Check sheet for the modelled part. Datum: model origin and axes. Units: mm. Face numbers are marked on the shaded views. A direction names the side the tool comes from. Coordinates: 2 decimals unless noted, no trailing zeros. Write each loop counter-clockwise with the first axis right and the second up, starting at its lowest first coordinate (ties: lowest second). Pieces come first, ordered by that corner, then holes. Notation, with made-up numbers: M 43.25,65 L 70.25,65 A15 ccw 70.25,75 Z; hole C 38,-5 d1. An arc over 180 degrees is marked long. Answer as CSV lines item,"result".
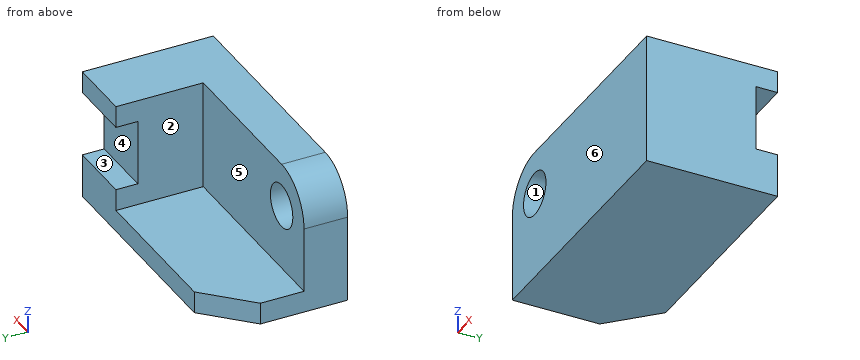
from build123d import *

# Parameters (mm, degrees)
SKETCH2_W           = 120
SKETCH2_H           = 60
BOSS_EXTRUDE1_DEPTH = 20
BOSS_EXTRUDE2_DEPTH = 40
FILLET1_R           = 20
CHAMFER1_SIZE       = 20
SKETCH8_W           = 30
SKETCH8_H           = 30
CUT_EXTRUDE1_DEPTH  = 10
SKETCH11_R          = 10
CUT_EXTRUDE3_DEPTH  = 141


with BuildPart() as part:
    # Sketch2 → Boss-Extrude1 (new body)
    with BuildSketch(Plane(origin=(0, 0, 0), x_dir=(1, 0, 0), z_dir=(0, 1, 0))):
        with Locations((-60, -30)):
            Rectangle(SKETCH2_W, SKETCH2_H)
    extrude(amount=-BOSS_EXTRUDE1_DEPTH)

    # Sketch3 → Boss-Extrude2 (add)
    with BuildSketch(Plane(origin=(0, 0, 0), x_dir=(1, 0, 0), z_dir=(0, 1, 0))):
        Polygon((-120, -10), (-30, -10), (-30, -60), (0, -60), (0, 0), (-120, 0), align=None)
    extrude(amount=BOSS_EXTRUDE2_DEPTH)

    # Fillet1
    fillet1_edges = [part.edges().sort_by_distance(p)[0] for p in [
        (-120, -10, 60),
    ]]
    fillet(fillet1_edges, radius=FILLET1_R)

    # Chamfer1
    chamfer1_edges = [part.edges().sort_by_distance(p)[0] for p in [
        (-120, 40, 5),
    ]]
    chamfer(chamfer1_edges, length=CHAMFER1_SIZE)

    # Sketch8 → Cut-Extrude1 (cut)
    with BuildSketch(Plane(origin=(0, 40, 0), x_dir=(1, 0, 0), z_dir=(0, 1, 0))):
        with Locations((-15, -35)):
            Rectangle(SKETCH8_W, SKETCH8_H)
    extrude(amount=-CUT_EXTRUDE1_DEPTH, mode=Mode.SUBTRACT)

    # Sketch11 → Cut-Extrude3 (cut, through all)
    with BuildSketch(Plane(origin=(0, 0, 0), x_dir=(1, 0, 0), z_dir=(0, 1, 0))):
        with Locations(Location((-100, -40, 0), (0, 0, 270))):
            Circle(SKETCH11_R)
    extrude(amount=-CUT_EXTRUDE3_DEPTH, mode=Mode.SUBTRACT)


solid = part.part
1) Section check C-C, the plane x = -15.5. Record the boundary of the cut face in (y, z), plus the area to 3 significant figures.
Answer key:
outline,"M -20,0 L 40,0 L 40,20 L 30,20 L 30,50 L 40,50 L 40,60 L -20,60 Z"
area,"3,300 mm2"
2) Mould release check, pull along X, two halves, no side actions. Record for the marked faces 1, 2 and 3: pulls with the +X half, pulls with the -X half, needs draft (parallel to the pull), parting line crosses it, or undercut.
Answer key:
face 1,"undercut"
face 2,"pulls with the -X half"
face 3,"needs draft"
3) Section check B-B, the plane z = 37. Record the boundary of the cut face in (x, y).
Answer key:
outline,"M -120,-20 L -109.54,-20 L -109.54,0 L -120,0 Z; M -90.46,-20 L 0,-20 L 0,30 L -30,30 L -30,0 L -90.46,0 Z"
4) Section check D-D, the plane y = -15. Record the boundary of the cut face in (x, z).
Answer key:
outline,"M -120,0 L 0,0 L 0,60 L -100,60 A20 ccw -120,40 Z; hole C -100,40 d20"
5) Section check A-A, the plane x = -94. Record the boundary of the cut face in (y, z).
Answer key:
outline,"M -20,0 L 40,0 L 40,10 L 0,10 L 0,32 L -20,32 Z; M -20,48 L 0,48 L 0,60 L -20,60 Z"
6) Depth check by flat-ended pin: P1, Ø3, axis at x = -19.5, y = 37, coming from the -Z side; P2, Ø6, axis at y = 17.5, z = 43.5, coming from the -X side; P3, Ø20, axis at x = -79.5, y = 15, coming from the +Z side; P4, Ø10, axis at y = 4.5, z = 51.5, coming from the -X side. Enter the tip coordinate at first touch or a pass-through.
Answer key:
P1,"stops at z = 0"
P2,"stops at x = -30"
P3,"stops at z = 10"
P4,"stops at x = -117.7"
7) Thickness scan on line 1 along X through (y, z) = (-11, 40); line 2 along Y through (x, z) = (-100, 52); line 3 along Z through (x, y) = (-63.5, 26.5). Record the ranges inside material, lowest first.
Answer key:
line 1,"x = -120 to -110, -90 to 0"
line 2,"y = -20 to 0"
line 3,"z = 0 to 10"
8) Tool access check on the marked faces 4, 5 and 6. Record the directions out of +Z, -Z, +X, -X, +Y, -Y that give a thin tool (end or side, any length) a straight path to the whole face; none if there is none.
Answer key:
face 4,"+X, -X, +Y"
face 5,"+Z, -X, +Y"
face 6,"+Z, -Z, +X, -X, -Y"
